Geometry check sheet. Reference: the model listing, model coordinates, mm. Round coordinates to 2 decimals unless told otherwise and drop trailing zeros. Write each loop counter-clockwise with the first axis right and the second up, starting at its lowest first coordinate (ties: lowest second). Pieces come first, ordered by that corner, then holes. Notation, with made-up numbers: (19.5, 49.5) - (59.5, 49.5) arc R21 cw to (59.5, 76.5) - close; hole circle Ø10 at (37, -28). An arc over 180 degrees is marked (long way). Return JSON: item names as keys, results as strings. Group by question number.
Autodesk Inventor part; units mm, degrees
ref_plane "YZ Plane" through (0, 0, 0) normal (1, 0, 0) x (0, 1, 0)
ref_plane "XZ Plane" through (0, 0, 0) normal (0, 1, 0) x (-1, 0, 0)
ref_plane "XY Plane" through (0, 0, 0) normal (0, 0, 1) x (1, 0, 0)
sketch "Sketch1" plane through (0, 0, 0) normal (0, 1, 0) x (-1, 0, 0)
  line L0 (1.5588, -12.1667) -> (-1.5588, -12.1667)
  line L1 (-1.5588, -12.1667) -> (-11.3161, 4.7333)
  line L2 (-11.3161, 4.7333) -> (-9.7572, 7.4333)
  line L3 (-9.7572, 7.4333) -> (9.7572, 7.4333)
  line L4 (9.7572, 7.4333) -> (11.3161, 4.7333)
  line L5 (11.3161, 4.7333) -> (1.5588, -12.1667)
  circle A0 centre (0, 0) radius 7.4333 construction
  line L6 (-1.5588, -12.1667) -> (-3.1177, -14.8667) construction
  line L7 (-3.1177, -14.8667) -> (-22.6321, -14.8667) construction
  line L8 (-22.6321, -14.8667) -> (-24.191, -12.1667) construction
  line L9 (-24.191, -12.1667) -> (-14.4338, 4.7333) construction
  line L10 (-14.4338, 4.7333) -> (-11.3161, 4.7333) construction
  dimension "d0" = 19.6
  dimension "d1" = 3.1177
  dimension "d4" = 14.8667
  dimension "d5" = 22.3
extrude "Extrusion1" add sketch "Sketch1" along normal mid plane 1.9
equation "\"d0\" = CouncilTriangleTrimmed"
equation "\"d5\" = CouncilTriangleHeight"
equation "\"CouncilTriangleHeight\" = 22.3"
equation "\"CouncilTriangleTrimmed\" = 19.6"
properties part number "FactionSpecial_Council_CommandToken_Single" material "ABS Plastic"
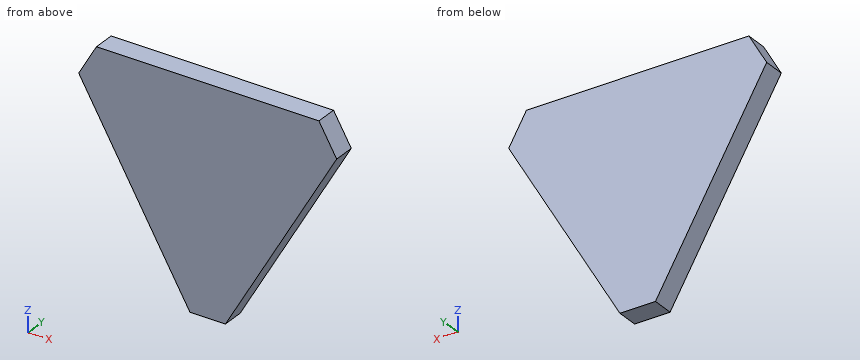
1. Section check B-B (z = -8.5). Enter the section's corners in (x, y).
2. Section check C-C (x = 4.25). Enter the section's corners in (y, z).
3. Material ranges on line 1 along X through (y, z) = (0.5, -6); line 2 along X through (y, z) = (0.75, -4.25); line 3 along Z through (x, y) = (-8.75, 0.2), recorded low to high.
4. Depth check by flat-ended pin: pin 1 Ø10 at (x, z) = (-8, -8) entering from -Y. Enter the tip coordinate at first touch or a pass-through.
5. Section check A-A (y = 0.55). Enter the section's corners in (x, z).
Result sheet:
{
 "1": {"outline": "(-3.68, -0.95) - (3.68, -0.95) - (3.68, 0.95) - (-3.68, 0.95) - close"},
 "2": {"outline": "(-0.95, -7.51) - (0.95, -7.51) - (0.95, 7.43) - (-0.95, 7.43) - close"},
 "3": {"line 1": "x = -5.12 to 5.12", "line 2": "x = -6.13 to 6.13", "line 3": "z = 0.29 to 7.43"},
 "4": {"pin 1": "stops at y = -0.95"},
 "5": {"outline": "(-11.32, 4.73) - (-1.56, -12.17) - (1.56, -12.17) - (11.32, 4.73) - (9.76, 7.43) - (-9.76, 7.43) - close"}
}
